```python
from build123d import *

# Parameters (mm, degrees)
SKETCH11_W          = 38.1
SKETCH11_H          = 38.1
SKETCH12_W          = 38.1
SKETCH12_H          = 38.1
BOSS_EXTRUDE5_DEPTH = 12.7
BOSS_EXTRUDE5_TAPER = 20
BOSS_EXTRUDE6_DEPTH = 38.1
SKETCH15_R          = 12.065
CUT_EXTRUDE3_DEPTH  = 25.4
SKETCH16_W          = 23.310601064
SKETCH16_H          = 76.2
CUT_EXTRUDE4_DEPTH  = 59.830675793
SKETCH17_R          = 7.62
BOSS_EXTRUDE7_DEPTH = 6.35
SKETCH18_R          = 5.08
BOSS_EXTRUDE8_DEPTH = 3.81
SKETCH19_R          = 3.1115
BOSS_EXTRUDE9_DEPTH = 7.62
FILLET2_R           = 5.08


with BuildPart() as part:
    # Sweep1: sweep along a path in Sketch10
    with BuildLine(Plane(origin=(0, 0, 0), x_dir=(0, 0, -1), z_dir=(1, 0, 0))) as sweep1_path:
        Line((0, 96.393), (0, -5.207))
        Line((0, -5.207), (-25.324322261, -30.531322261))
    # Sketch11 → Sweep1 (sweep)
    with BuildSketch(Plane(origin=(0, 96.393, 0), x_dir=(1, 0, 0), z_dir=(0, 1, 0))):
        Rectangle(SKETCH11_W, SKETCH11_H)
    sweep(path=sweep1_path.line, transition=Transition.RIGHT)

    # Sketch12 → Boss-Extrude5 (add)
    with BuildSketch(Plane(origin=(0, -27.927822261, 27.927822261), x_dir=(1, 0, 0), z_dir=(0, -0.7071067811865461, 0.7071067811865489))):
        with Locations((0, -3.68190501)):
            Rectangle(SKETCH12_W, SKETCH12_H)
    extrude(amount=BOSS_EXTRUDE5_DEPTH, taper=BOSS_EXTRUDE5_TAPER)

    # Sketch13 → Boss-Extrude6 (add)
    with BuildSketch(Plane(origin=(0, 0, -19.05), x_dir=(-1, 0, 0), z_dir=(0, 0, -1))):
        with BuildLine():
            Line((-19.05, 96.393), (19.05, 96.393))
            ThreePointArc((19.05, 96.393), (0, 115.443), (-19.05, 96.393))
        make_face()
    extrude(amount=-BOSS_EXTRUDE6_DEPTH)

    # Sketch15 → Cut-Extrude3 (cut)
    with BuildSketch(Plane(origin=(0, -36.908078382, 36.908078382), x_dir=(1, 0, 0), z_dir=(0, -0.7071067811865461, 0.7071067811865489))):
        with Locations(Location((0, -3.68190501, 0), (0, 0, 270))):
            Circle(SKETCH15_R)
    extrude(amount=-CUT_EXTRUDE3_DEPTH, mode=Mode.SUBTRACT)

    # Sketch16 → Cut-Extrude4 (cut)
    with BuildSketch(Plane(origin=(19.05, 0, 0), x_dir=(0, 0, -1), z_dir=(1, 0, 0))):
        with Locations((0, 45.72)):
            Rectangle(SKETCH16_W, SKETCH16_H)
    extrude(amount=-CUT_EXTRUDE4_DEPTH, mode=Mode.SUBTRACT)

    # Sketch17 → Boss-Extrude7 (add)
    with BuildSketch(Plane.XY.offset(19.05)):
        with Locations(Location((0, 96.393, 0), (0, 0, 90))):
            Circle(SKETCH17_R)
    extrude(amount=BOSS_EXTRUDE7_DEPTH)

    # Sketch18 → Boss-Extrude8 (add)
    with BuildSketch(Plane.XY.offset(25.4)):
        with Locations(Location((0, 96.393, 0), (0, 0, 180))):
            Circle(SKETCH18_R)
    extrude(amount=BOSS_EXTRUDE8_DEPTH)

    # Sketch19 → Boss-Extrude9 (add)
    with BuildSketch(Plane.XY.offset(29.21)):
        with Locations(Location((0, 96.393, 0), (0, 0, 180))):
            Circle(SKETCH19_R)
    extrude(amount=BOSS_EXTRUDE9_DEPTH)

    # Fillet2
    # the kernel refuses this fillet: 5.08 mm, written as the material it takes off along each edge
    with BuildSketch(Plane(origin=(19.05, 96.393, 19.05), x_dir=(-1, 0, 0), z_dir=(0, -1, 0))) as fillet2_piece_1_section:
        with BuildLine():
            CenterArc((FILLET2_R, FILLET2_R), FILLET2_R, 180, 90)
            Line((0, FILLET2_R), (0, 0))
            Line((0, 0), (FILLET2_R, 0))
        make_face()
    fillet2_piece_1 = extrude(amount=106.409231637, mode=Mode.PRIVATE)
    fillet2_piece_1 = split(fillet2_piece_1, bisect_by=Plane(origin=(17.892257619, 26.96392305, -5.230154687), z_dir=(0, 0.7071067811865489, 0.7071067811865462)), keep=Keep.TOP, mode=Mode.PRIVATE)
    add(fillet2_piece_1, mode=Mode.SUBTRACT)
    with BuildSketch(Plane(origin=(19.05, 96.393, -19.05), x_dir=(0, 0, 1), z_dir=(0, -1, 0))) as fillet2_piece_2:
        with BuildLine():
            CenterArc((FILLET2_R, FILLET2_R), FILLET2_R, 180, 90)
            Line((0, FILLET2_R), (0, 0))
            Line((0, 0), (FILLET2_R, 0))
        make_face()
    extrude(amount=122.190768363, mode=Mode.SUBTRACT)
    with BuildSketch(Plane(origin=(19.05, 11.664024484, 10.069743879), x_dir=(-1, 0, 0), z_dir=(0, -0.7071067811865462, 0.7071067811865489))) as fillet2_piece_3_section:
        with BuildLine():
            CenterArc((FILLET2_R, FILLET2_R), FILLET2_R, 180, 90)
            Line((0, FILLET2_R), (0, 0))
            Line((0, 0), (FILLET2_R, 0))
        make_face()
    fillet2_piece_3 = extrude(amount=53.323231637, mode=Mode.PRIVATE)
    fillet2_piece_3 = split(fillet2_piece_3, bisect_by=Plane(origin=(17.881962417, -12.866336341, 19.05), z_dir=(0, 0, 1)), keep=Keep.TOP, mode=Mode.PRIVATE)
    add(fillet2_piece_3, mode=Mode.SUBTRACT)
    with BuildSketch(Plane(origin=(19.05, -4.117512242, -28.030256121), x_dir=(0, 0.7071067811865489, 0.7071067811865462), z_dir=(0, -0.7071067811865462, 0.7071067811865489))) as fillet2_piece_4:
        with BuildLine():
            CenterArc((FILLET2_R, FILLET2_R), FILLET2_R, 180, 90)
            Line((0, FILLET2_R), (0, 0))
            Line((0, 0), (FILLET2_R, 0))
        make_face()
    extrude(amount=69.104768363, mode=Mode.SUBTRACT)
    with BuildSketch(Plane(origin=(-19.05, -4.117512242, -28.030256121), x_dir=(0, 0.7071067811865488, 0.7071067811865461), z_dir=(0, -0.7071067811865462, 0.7071067811865489))) as fillet2_piece_5:
        with BuildLine():
            CenterArc((FILLET2_R, -FILLET2_R), FILLET2_R, 90, 90)
            Line((0, -FILLET2_R), (0, 0))
            Line((0, 0), (FILLET2_R, 0))
        make_face()
    extrude(amount=69.104768363, mode=Mode.SUBTRACT)
    with BuildSketch(Plane(origin=(-19.05, 11.664024484, 10.069743879), x_dir=(0, -0.7071067811865489, -0.7071067811865462), z_dir=(0, -0.7071067811865462, 0.7071067811865489))) as fillet2_piece_6_section:
        with BuildLine():
            CenterArc((FILLET2_R, FILLET2_R), FILLET2_R, 180, 90)
            Line((0, FILLET2_R), (0, 0))
            Line((0, 0), (FILLET2_R, 0))
        make_face()
    fillet2_piece_6 = extrude(amount=53.323231637, mode=Mode.PRIVATE)
    fillet2_piece_6 = split(fillet2_piece_6, bisect_by=Plane(origin=(-17.881962417, -12.866336341, 19.05), z_dir=(0, 0, 1)), keep=Keep.TOP, mode=Mode.PRIVATE)
    add(fillet2_piece_6, mode=Mode.SUBTRACT)
    with BuildSketch(Plane(origin=(19.05, -15.477476632, 40.378167891), x_dir=(0, 0.7071067811865461, -0.7071067811865488), z_dir=(0, -0.7071067811865489, -0.7071067811865462)), Plane(origin=(-19.05, -45.585167891, 10.270476632), x_dir=(0, 0.7071067811865461, -0.7071067811865489), z_dir=(0, 0.7071067811865489, 0.7071067811865462))) as fillet2_piece_7:
        with BuildLine():
            CenterArc((FILLET2_R * 0.176326980708, -FILLET2_R), FILLET2_R, 90, 20)
            Line((-FILLET2_R * 0.165693162617, -FILLET2_R * 0.0603073792141), (0, 0))
            Line((0, 0), (FILLET2_R * 0.176326980708, 0))
        make_face()
    extrude(amount=42.57870531, mode=Mode.SUBTRACT)
    with BuildSketch(Plane(origin=(-19.05, 96.393, -19.05), x_dir=(0, 0, 1), z_dir=(0, -1, 0))) as fillet2_piece_8:
        with BuildLine():
            CenterArc((FILLET2_R, -FILLET2_R), FILLET2_R, 90, 90)
            Line((0, -FILLET2_R), (0, 0))
            Line((0, 0), (FILLET2_R, 0))
        make_face()
    extrude(amount=122.190768363, mode=Mode.SUBTRACT)
    with BuildSketch(Plane(origin=(-19.05, 96.393, 19.05), x_dir=(1, 0, 0), z_dir=(0, -1, 0))) as fillet2_piece_9_section:
        with BuildLine():
            CenterArc((FILLET2_R, -FILLET2_R), FILLET2_R, 90, 90)
            Line((0, -FILLET2_R), (0, 0))
            Line((0, 0), (FILLET2_R, 0))
        make_face()
    fillet2_piece_9 = extrude(amount=106.409231637, mode=Mode.PRIVATE)
    fillet2_piece_9 = split(fillet2_piece_9, bisect_by=Plane(origin=(-17.892257619, 26.96392305, -5.230154687), z_dir=(0, 0.7071067811865489, 0.7071067811865462)), keep=Keep.TOP, mode=Mode.PRIVATE)
    add(fillet2_piece_9, mode=Mode.SUBTRACT)
    with BuildSketch(Plane(origin=(0, 96.393, -19.05), x_dir=(-1, 0, 0), z_dir=(0, -1, 0))) as fillet2_piece_10:
        with BuildLine():
            CenterArc((19.05 - FILLET2_R, -FILLET2_R), FILLET2_R, 0, 90)
            Line((19.05 - FILLET2_R, 0), (19.05, 0))
            Line((19.05, 0), (19.05, -FILLET2_R))
        make_face()
    revolve(axis=Axis((0, 96.393, -19.05), (0, 0, -1)), revolution_arc=180, mode=Mode.SUBTRACT)
    with BuildSketch(Plane(origin=(0, 96.393, 19.05), x_dir=(-1, 0, 0), z_dir=(0, -1, 0))) as fillet2_piece_11:
        with BuildLine():
            CenterArc((19.05 - FILLET2_R, FILLET2_R), FILLET2_R, 270, 90)
            Line((19.05, FILLET2_R), (19.05, 0))
            Line((19.05, 0), (19.05 - FILLET2_R, 0))
        make_face()
    revolve(axis=Axis((0, 96.393, 19.05), (0, 0, -1)), revolution_arc=180, mode=Mode.SUBTRACT)
    with BuildSketch(Plane(origin=(19.05, 96.393, 19.05), x_dir=(-1, 0, 0), z_dir=(0, -1, 0))) as fillet2_piece_12a_section:
        with BuildLine():
            CenterArc((FILLET2_R, FILLET2_R), FILLET2_R, 180, 90)
            Line((0, FILLET2_R), (0, 0))
            Line((0, 0), (FILLET2_R, 0))
        make_face()
    fillet2_piece_12a = extrude(amount=106.409231637, mode=Mode.PRIVATE)
    fillet2_piece_12a = split(fillet2_piece_12a, bisect_by=Plane(origin=(17.951071981, 0.436282509, 21.297485854), z_dir=(0, -0.7071067811865489, -0.7071067811865462)), keep=Keep.TOP, mode=Mode.PRIVATE)
    with BuildSketch(Plane(origin=(19.05, 11.664024484, 10.069743879), x_dir=(-1, 0, 0), z_dir=(0, -0.7071067811865462, 0.7071067811865489))) as fillet2_piece_12b_section:
        with BuildLine():
            CenterArc((FILLET2_R, FILLET2_R), FILLET2_R, 180, 90)
            Line((0, FILLET2_R), (0, 0))
            Line((0, 0), (FILLET2_R, 0))
        make_face()
    fillet2_piece_12b = extrude(amount=53.323231637, mode=Mode.PRIVATE)
    fillet2_piece_12b = split(fillet2_piece_12b, bisect_by=Plane(origin=(17.951071981, 5.862193339, 19.05), z_dir=(0, 0, -1)), keep=Keep.TOP, mode=Mode.PRIVATE)
    fillet2_piece_12 = fillet2_piece_12a & fillet2_piece_12b
    add(fillet2_piece_12, mode=Mode.SUBTRACT)
    with BuildSketch(Plane(origin=(-19.05, 96.393, 19.05), x_dir=(1, 0, 0), z_dir=(0, -1, 0))) as fillet2_piece_13a_section:
        with BuildLine():
            CenterArc((FILLET2_R, -FILLET2_R), FILLET2_R, 90, 90)
            Line((0, -FILLET2_R), (0, 0))
            Line((0, 0), (FILLET2_R, 0))
        make_face()
    fillet2_piece_13a = extrude(amount=106.409231637, mode=Mode.PRIVATE)
    fillet2_piece_13a = split(fillet2_piece_13a, bisect_by=Plane(origin=(-17.951071981, 0.436282509, 21.297485854), z_dir=(0, -0.7071067811865489, -0.7071067811865462)), keep=Keep.TOP, mode=Mode.PRIVATE)
    with BuildSketch(Plane(origin=(-19.05, 11.664024484, 10.069743879), x_dir=(0, -0.7071067811865489, -0.7071067811865462), z_dir=(0, -0.7071067811865462, 0.7071067811865489))) as fillet2_piece_13b_section:
        with BuildLine():
            CenterArc((FILLET2_R, FILLET2_R), FILLET2_R, 180, 90)
            Line((0, FILLET2_R), (0, 0))
            Line((0, 0), (FILLET2_R, 0))
        make_face()
    fillet2_piece_13b = extrude(amount=53.323231637, mode=Mode.PRIVATE)
    fillet2_piece_13b = split(fillet2_piece_13b, bisect_by=Plane(origin=(-17.951071981, 5.862193339, 19.05), z_dir=(0, 0, -1)), keep=Keep.TOP, mode=Mode.PRIVATE)
    fillet2_piece_13 = fillet2_piece_13a & fillet2_piece_13b
    add(fillet2_piece_13, mode=Mode.SUBTRACT)


solid = part.part
```
Design review of the part built by this model. Coordinates are the model's own, in mm. A direction names the side the tool comes from. Coordinates: 2 decimals unless noted, no trailing zeros. Order: outer loops, then holes, each group sorted by start corner. A loop starts at its lowest first (then second) coordinate and runs counter-clockwise, first axis right, second up. Notation, with made-up numbers: (20, 78.5) - (60, 78.5) arc R10 ccw to (60, 85.5) - close; hole circle Ø5 at (62, 27). An arc over 180 degrees is marked (long way). Answer in a Markdown table with one row per item.
(1) Consider section A-A on y = 39. State the section outline as (x, z) points, plus the area to 3 significant figures.
Checked values:
| item | result |
|---|---|
| outline | (-19.05, -13.97) arc R5.08 ccw to (-13.97, -19.05) - (13.97, -19.05) arc R5.08 ccw to (19.05, -13.97) - (19.05, -11.66) - (-19.05, -11.66) - close; (-19.05, 11.66) - (19.05, 11.66) - (19.05, 13.97) arc R5.08 ccw to (13.97, 19.05) - (-13.97, 19.05) arc R5.08 ccw to (-19.05, 13.97) - close |
| area | 541 mm^2 |
(2) For faces 4 (the flat face through (-19.05, 13, 12)), 5 (the flat face through (5, 98, 25.4)), 6 (the flat face through (0, 96, 36.83)), 7 (the flat face through (0, 83.82, 0)), list the 3-axis set-ups (+Z, -Z, +X, -X, +Y, -Y) from which the entire face can be reached by the end or side of a thin tool; tool diameter is ignored.
Checked values:
| item | result |
|---|---|
| face 4 | +Z, -Z, -X, +Y, -Y |
| face 5 | +Z |
| face 6 | +Z, +X, -X, +Y |
| face 7 | +X, -X |
(3) The part is to be moulded in two halves that separate along Y. For faces 1 (the flat face through (-16.616, -35.434, 29.879)), 2 (the flat face through (0, 49, -19.05)), 3 (the cylindrical face through (-1.44, 99.15, 32.97)), say which applies: released by +Y, released by -Y, zero draft, split by the parting line, or undercut.
Checked values:
| item | result |
|---|---|
| face 1 | released by -Y |
| face 2 | zero draft |
| face 3 | undercut |
(4) Clearance check with flat-ended pins moving along their axes: pin 1 (1.5 mm diameter, centred on x = -1, z = 37.5, fed in from -Y); pin 2 (10 mm diameter, centred on x = -12.5, y = -27.5, fed in from -Z); pin 3 (2 mm diameter, centred on x = -13, z = 14, fed in from +Y). State where each tip first meets the part, or that it passes through.
Checked values:
| item | result |
|---|---|
| pin 1 | y = -26.46 |
| pin 2 | z = -9.65 |
| pin 3 | y = 111.19 |
(5) Wall thickness on line 1 along Z through (x, y) = (-10, 21); line 2 along Y through (x, z) = (2.5, 19.5); line 3 along X through (y, z) = (-26, 19.5): over which ranges is each line inside the solid? List them lowest first. Write a range as from..to.
Checked values:
| item | result |
|---|---|
| line 1 | -19.05..-11.66, 11.66..19.05 |
| line 2 | -47.57..-41.4, -18.4..2.23, 89.19..103.59 |
| line 3 | -19.05..-12.03, 12.03..19.05 |
